from build123d import *

# Parameters (mm, degrees)
F0_R     = 4.7625
F1_DEPTH = 6.35


with BuildPart() as f1:
    # F0 (on Front) → F1 (new body)
    with BuildSketch(Plane.XZ):
        with BuildLine():
            ThreePointArc((3.175, -19.05), (9.910192, -16.260192), (12.7, -9.525))
            Line((12.7, -9.525), (12.7, 112.161003))
            Line((12.7, 112.161003), (-12.7, 112.161003))
            Line((-12.7, 112.161003), (-12.7, -9.525))
            ThreePointArc((-12.7, -9.525), (-9.910192, -16.260192), (-3.175, -19.05))
            Line((-3.175, -19.05), (3.175, -19.05))
        make_face()
        Circle(F0_R, mode=Mode.SUBTRACT)
        with Locations((0, 76.962)):
            Circle(F0_R, mode=Mode.SUBTRACT)
    extrude(amount=F1_DEPTH)


solid = f1.part
CAD build for the part. Positions are in the model's coordinates, mm. Coordinates: 2 decimals unless noted, no trailing zeros. Loops run counter-clockwise (first coordinate to the right, second up) from the corner with the lowest first, then second, coordinate; pieces in that order, holes last. Notation, with made-up numbers: (-10, -38) - (20, -38) arc R19 ccw to (20, -3) - close; hole circle Ø1 at (56, -35). An arc over 180 degrees is marked (long way). Use one line per item in the form item = value. Start each with the question number.
1) Band-saw the part on A-A (x = 0). Give the cut face in (y, z).
2) Drill centre lines: L1, parallel to Z at x = 0.5, y = -4.75; L2, parallel to Z at x = 0, y = -2.75; L3, parallel to X at y = -5.5, z = -10. Where is each one in solid material? Low to high. Write a range as from..to.
3) Band-saw the part on C-C (y = -3.25). State how many separate pieces and enclosed holes the cut face has, and give its area (3 significant figures).
4) Two-plate mould, pull along X, no slides. Class faces 1 (the face through (-3.78, -3.13, -2.9)), 2 (the face through (-12.7, -3, 52)), 3 (the face through (0, -6.35, 47)): +X half, -X half, draft (parallel to the pull), parting line (faces both ways), or undercut.
5) Flat gauge pin, fed straight in: pin 1 (6 mm diameter, centred on x = -9, z = 35.5, fed in from +Y). Where does the tip first touch, or does it go through?
6) Band-saw the part on B-B (z = 0). Give the cut face in (x, y), and give its area (3 significant figures).
Check values:
q1.outline = (-6.35, -19.05) - (0, -19.05) - (0, -4.76) - (-6.35, -4.76) - close; (-6.35, 4.76) - (0, 4.76) - (0, 72.2) - (-6.35, 72.2) - close; (-6.35, 81.72) - (0, 81.72) - (0, 112.16) - (-6.35, 112.16) - close
q2.L1 = -19.05..-4.74, 4.74..72.23, 81.7..112.16
q2.L2 = -19.05..-4.76, 4.76..72.2, 81.72..112.16
q2.L3 = -12.69..12.69
q3.separate_pieces = 1
q3.enclosed_holes = 2
q3.area = 3,150 mm2
q4.face_1 = undercut
q4.face_2 = -X half
q4.face_3 = draft
q5.pin_1 = 0
q6.outline = (-12.7, -6.35) - (-4.76, -6.35) - (-4.76, 0) - (-12.7, 0) - close; (4.76, -6.35) - (12.7, -6.35) - (12.7, 0) - (4.76, 0) - close
q6.area = 101 mm2
